from build123d import *

# Parameters (mm, degrees)
F1_DEPTH = 1.5
F2_R     = 10
F3_R     = 20


with BuildPart() as f1:
    # F0 (on Top) → F1 (new body)
    with BuildSketch(Plane.XY):
        with BuildLine():
            Line((0, 36.5856099731), (0, 196.5856099731))
            ThreePointArc((0, 196.5856099731), (-307.3351576975, 315.2560594706), (-635, 349.5099039223))
            Line((-635, 349.5099039223), (-621.0269461922, 189.7971680702))
            Line((-621.0269461922, 189.7971680702), (-361.6779078132, 171.4103170113))
            Line((-361.6779078132, 171.4103170113), (-225.8692382849, 137.4102393502))
            Line((-225.8692382849, 137.4102393502), (0, 36.5856099731))
        make_face()
    extrude(amount=F1_DEPTH)

    # F2
    f2_edges = [f1.edges().sort_by_distance(p)[0] for p in [
        (0, 196.58561, 0.75),
        (-635, 349.509904, 0.75),
        (-621.026946, 189.797168, 0.75),
        (0, 36.58561, 0.75),
    ]]
    fillet(f2_edges, radius=F2_R)

    # F3
    f3_edges = [f1.edges().sort_by_distance(p)[0] for p in [
        (-361.677908, 171.410317, 0.75),
        (-225.869238, 137.410239, 0.75),
    ]]
    fillet(f3_edges, radius=F3_R)


solid = f1.part
Verification items for the finished model (mm, model axes). Give positions to 0.01 mm unless a question says otherwise; leave off trailing zeros. Loops run counter-clockwise (first coordinate to the right, second up) from the corner with the lowest first, then second, coordinate; pieces in that order, holes last.
1) Sectioned sample at B-B, the plane x = -582. Enter the section's corners in (y, z), then the cut area to 3 significant figures.
2) Thickness scan on line 1 along Y through (x, z) = (-348.5, 0.65); line 2 along Y through (x, z) = (-185, 1.35); line 3 along X through (y, z) = (94, 0.2). Record the ranges inside material, lowest first.
3) Sectioned sample at A-A, the plane z = 0.95. Enter the section's corners in (x, y).
4) Sectioned sample at C-C, the plane y = 220.5. Enter the section's corners in (x, z).
Answers:
1. outline: (187.03, 0) - (349.87, 0) - (349.87, 1.5) - (187.03, 1.5) - close
1. area: 244 mm2
2. line 1: y = 168.11 to 324.44
2. line 2: y = 119.17 to 279.1
2. line 3: x = -128.62 to 0
3. outline: (-634.07, 338.89) - (-621.77, 198.3) arc R10 ccw to (-612.52, 189.19) - (-363.42, 171.53) arc R20 cw to (-359.98, 170.99) - (-227.57, 137.84) arc R20 cw to (-224.27, 136.7) - (-14.08, 42.87) arc R10 ccw to (0, 52) - (0, 190.64) arc R10 ccw to (-5.24, 199.44) arc R1250 ccw to (-624.3, 349.76) arc R10 ccw to start
4. outline: (-623.71, 0) - (-45.94, 0) - (-45.94, 1.5) - (-623.71, 1.5) - close
